Here's how the part is built. I have some questions about the finished solid (model axes, mm). A direction names the side the tool comes from. Round coordinates to 2 decimals unless told otherwise and drop trailing zeros. Order: outer loops, then holes, each group sorted by start corner. A loop starts at its lowest first (then second) coordinate and runs counter-clockwise, first axis right, second up. Notation, with made-up numbers: (65.5, -5) -> (84.5, -5) arc R32 cw to (84.5, 31) -> close; hole circle Ø6 at (83, -21.75). An arc over 180 degrees is marked (long way). One line per item, written item: value.
Autodesk Inventor part; units mm, degrees
ref_plane "Plan de construction1" through (0, 5, 0) normal (0, -1, 0) x (1, 0, 0)
ref_plane "YZ Plane" through (0, 0, 0) normal (1, 0, 0) x (0, 1, 0)
ref_plane "XZ Plane" through (0, 0, 0) normal (0, 1, 0) x (-1, 0, 0)
sketch "Esquisse1" plane through (0, 0, 0) normal (0, 1, 0) x (-1, 0, 0)
  circle A0 centre (0, 0) radius 17.75
  dimension "d0" = 35.5
extrude "Extrusion1" add sketch "Esquisse1" along normal blind 8
ref_plane "Plan de construction1" through (0, 5, 0) normal (0, -1, 0) x (1, 0, 0)
sketch "Esquisse2" plane through (0, 5, 0) normal (0, -1, 0) x (1, 0, 0)
  circle A0 centre (0, 0) radius 17.75 construction
  line L0 (0, 0) -> (11, 0) construction
  circle A1 centre (11, 0) radius 1.65
  dimension "d4" = 11
  dimension "d5" = 3.3
extrude "Extrusion2" cut sketch "Esquisse2" along normal through all both and the other way through all
sketch "Esquisse3" plane through (0, 5, 0) normal (0, -1, 0) x (1, 0, 0)
  line L0 (23.2, 2.825) -> (8.2, 2.825)
  line L1 (8.2, 2.825) -> (8.2, -2.825)
  line L2 (8.2, -2.825) -> (23.2, -2.825)
  line L3 (23.2, -2.825) -> (23.2, 2.825)
  circle A0 centre (11, 0) radius 1.65 construction
  circle A1 centre (0, 0) radius 17.75 construction
  line L4 (0, 0) -> (8.2, 0) construction
  dimension "d8" = 5.65
  dimension "d9" = 2.8
  dimension "d10" = 15
extrude "Extrusion3" cut sketch "Esquisse3" along normal blind 2.3
pattern_circular "Réseau circulaire1" count 3 over 360 about axis through (0, 0, 0) along (0, -1, 0) of "Extrusion3", "Extrusion2"
ref_plane "Work Plane2" through (0, 6.5, 0) normal (0, 1, 0) x (1, 0, 0)
sketch "Sketch4" plane through (0, 6.5, 0) normal (0, 1, 0) x (1, 0, 0)
  circle A0 centre (0, 0) radius 17
  circle A1 centre (-5.5, -9.5263) radius 1.65
  circle A2 centre (11, 0) radius 1.65
  circle A3 centre (0, 0) radius 17.75
  circle A4 centre (0, 0) radius 17.75
  line L0 (-5.1051, -17) -> (-5.1051, 17)
  dimension "d17" = 34
extrude "Extrusion4" [suppressed]
sketch "Sketch7" plane through (0, 0, 0) normal (0, -1, 0) x (1, 0, 0)
  circle A0 centre (-5.5, -9.5263) radius 1.65
  circle A1 centre (-5.5, 9.5263) radius 1.65
  circle A2 centre (11, 0) radius 1.65
  circle A3 centre (0, 0) radius 17.75
  arc A4 (12.2653, -21.0869) -> (-1.702, -23.304) centre (6.3902, -29.1791) ccw construction
  line L0 (12.2653, -21.0869) -> (14.1974, -23.6673) construction
  arc A5 (16.0148, -22.871) -> (19.1393, -21.699) centre (17.1898, -21.2525) ccw construction
  arc A6 (19.1393, -21.699) -> (17.9505, 23.1047) centre (-68.5898, -1.6093) ccw construction
  arc A7 (17.9505, 23.1047) -> (14.8221, 24.7813) centre (15.9506, 23.1301) ccw construction
  line L1 (14.8221, 24.7813) -> (14.299, 23.7665) construction
  circle A8 centre (10.9719, 0.0309) radius 1.5
  circle A9 centre (12.314, 17.2549) radius 1.5
  circle A10 centre (12.3141, -17.2245) radius 1.5
  circle A11 centre (10.9719, -0.0082) radius 3
  circle A12 centre (10.9719, -0.0082) radius 1.5
  circle A13 centre (12.3141, -17.2245) radius 1.5
  circle A14 centre (12.3141, -17.2245) radius 1.5
  arc A15 (14.1974, -23.6673) -> (17.3392, -3.7967) centre (-72.5704, 0.2356) ccw
  arc A16 (17.3635, 3.6841) -> (14.299, 23.7665) centre (-72.5704, 0.2356) ccw
  circle A17 centre (0, 0) radius 17.75
  arc A18 (14.1974, -23.6673) -> (-0.0039, -17.75) centre (-0.0039, -37.75) ccw
  arc A19 (0, 17.75) -> (14.299, 23.7665) centre (0, 37.75) ccw
  circle A20 centre (-5.5, -9.5263) radius 1.65
  circle A21 centre (-5.5, 9.5263) radius 1.65
  circle A22 centre (11, 0) radius 1.65
  circle A23 centre (0, 0) radius 17.75
  dimension "d50" = 1.3141
  dimension "d51" = 17.2245
  dimension "d53" = 20
  dimension "d54" = 20
  dimension "d61" = 1.314
  dimension "d62" = 17.224
  dimension "d63" = 90
  dimension "d64" = 90
  dimension "d66" = 20
  dimension "d67" = 20
extrude "Extrusion5" add sketch "Sketch7" against normal blind 8 contours A3 A19 A16 | A15 A18 A3
sketch "Sketch8" plane through (0, 8, 0) normal (0, 1, 0) x (1, 0, 0)
  circle A0 centre (12.3141, 17.2245) radius 1.5
  circle A1 centre (12.314, -17.2549) radius 1.5
  circle A2 centre (-5.5, 9.5263) radius 1.65
  circle A3 centre (-5.5, -9.5263) radius 1.65
  circle A4 centre (11, 0) radius 1.65
  arc A5 (-0.0039, 17.75) -> (0, -17.75) centre (0, 0) ccw
  arc A6 (14.299, -23.7665) -> (0, -17.75) centre (0, -37.75) ccw
  arc A7 (14.299, -23.7665) -> (17.3635, -3.6841) centre (-72.5704, -0.2356) ccw
  arc A8 (17.3635, -3.6841) -> (17.3392, 3.7967) centre (0, 0) ccw
  arc A9 (17.3392, 3.7967) -> (14.1974, 23.6673) centre (-72.5704, -0.2356) ccw
  arc A10 (-0.0039, 17.75) -> (14.1974, 23.6673) centre (-0.0039, 37.75) ccw
  arc A11 (14.299, -23.7665) -> (0, -17.75) centre (0, -37.75) ccw
  arc A12 (14.8721, -21.5382) -> (13.3292, -20.2477) centre (0, -37.75) ccw
  arc A13 (12.6827, -1.3087) -> (12.7364, 0.5886) centre (0, 0) ccw
  arc A14 (10.3425, 14.4255) -> (10.6571, 14.5677) centre (-0.0039, 37.75) ccw
  arc A15 (15.5707, -3.4578) -> (15.5479, 3.5588) centre (0, 0) ccw
  arc A16 (15.5479, 3.5588) -> (13.2545, 20.0947) centre (-72.5704, -0.2356) ccw
  arc A17 (17.3392, 3.7967) -> (14.1974, 23.6673) centre (-72.5704, -0.2356) ccw
  arc A18 (13.3292, -20.2477) -> (15.5707, -3.4578) centre (-72.5704, -0.2356) ccw
  arc A19 (11.9075, 19.0825) -> (11.9222, 19.0926) centre (-0.6265, 37.1628) ccw
  arc A20 (13.2545, 20.0947) -> (14.7767, 21.4548) centre (-0.6265, 37.1628) ccw
  dimension "d59" = 2
  dimension "d68" = 1.8
  dimension "d69" = 1.8
ref_plane "Work Plane3" through (0, 6.5, 0) normal (0, 1, 0) x (1, 0, 0)
ref_plane "Work Plane4" through (0, 1.5, 0) normal (0, -1, 0) x (1, 0, 0)
extrude "Extrusion6" cut sketch "Sketch8" against normal up to surface (5 mm away) from surface at -1.5 contours A9 A8 A7 A12 A18 A15 A16 A20
equation "\"d6\" = d5"
properties part number "capacitor_glue"
Q1. I want a section at D-D on x = 4.5. Write out the boundary of the cut face in (y, z), then the cut area to 3 significant figures.
Answers:
outline: (0, -18.26) -> (8, -18.26) -> (8, 18.26) -> (0, 18.26) -> close
area: 292 mm2
Q2. Which directions (+Z, -Z, +X, -X, +Y, -Y) give clear straight access to the entire face, cutting with the end or side of a thin tool? Please do faces 4 (the face through (-4.02, 3.87, -12.61)), 5 (the face through (14.84, 4.04, 12.02)), 6 (the face through (0, 8, 0)).
Answers:
face 4: none
face 5: +X
face 6: +Z, -Z, +X, -X, +Y
Q3. I want a section at A-A on x = -5.5. Write out the boundary of the cut face in (y, z), then the cut area to 3 significant figures.
Answers:
outline: (0, -16.88) -> (8, -16.88) -> (8, -11.18) -> (5, -11.18) -> (5, -15.18) -> (2.7, -15.18) -> (2.7, -11.18) -> (0, -11.18) -> close; (0, -7.88) -> (2.7, -7.88) -> (2.7, -6.29) -> (5, -6.29) -> (5, -7.88) -> (8, -7.88) -> (8, 7.88) -> (5, 7.88) -> (5, 6.29) -> (2.7, 6.29) -> (2.7, 7.88) -> (0, 7.88) -> close; (0, 11.18) -> (2.7, 11.18) -> (2.7, 15.18) -> (5, 15.18) -> (5, 11.18) -> (8, 11.18) -> (8, 16.88) -> (0, 16.88) -> close
area: 192 mm2
Q4. For P1, Ø1, axis at y = 3, z = 15, coming from the -X side; P2, Ø0.7, axis at x = 13, y = 4.5, coming from the -Z side; P3, Ø2, axis at y = 4.5, z = 5, coming from the -X side, each with a flat end and sliding along its axis, tell me the tip position at first contact or that it passes through.
Answers:
P1: x = -10.09
P2: z = -22.86
P3: x = -17.29
Q5. If we mould it in two halves opening along X, with no side actions, what happens to faces 1 (the face through (13.006, 3.944, -18.555)), 2 (the face through (8.2, 4, 0)), 3 (the face through (12, 4, -2.825))? For each: pulls with the +X half, pulls with the -X half, needs draft (parallel to the pull), parting line crosses it, or undercut.
Answers:
face 1: undercut
face 2: pulls with the +X half
face 3: needs draft
Q6. I want a section at C-C on x = -10. Write out the boundary of the cut face in (y, z) (1 decimal).
Answers:
outline: (0, -14.7) -> (2.7, -14.7) -> (2.7, -11.7) -> (5, -11.7) -> (5, -14.7) -> (8, -14.7) -> (8, 14.7) -> (5, 14.7) -> (5, 11.7) -> (2.7, 11.7) -> (2.7, 14.7) -> (0, 14.7) -> close
Q7. I need wall thicknesses on line 1 along Y through (x, z) = (14.5, 1.5); line 2 along Z through (x, y) = (11.5, 2.75) (3 decimals); line 3 along Z through (x, y) = (-5.5, 2). Which ranges of each line are inside material? Lowest first, please.
Answers:
line 1: 0 to 2.7, 5 to 8
line 2: -21.39 to -18.484, -15.965 to -2.825, 2.825 to 15.995, 18.515 to 21.387
line 3: -16.88 to -11.18, -7.88 to 7.88, 11.18 to 16.88
Q8. I want a section at B-B on y = 5.5. Give the number of separate pieces and of enclosed holes in the cut face, then the cut area to 3 significant figures.
Answers:
separate pieces: 1
enclosed holes: 5
area: 1,040 mm2
